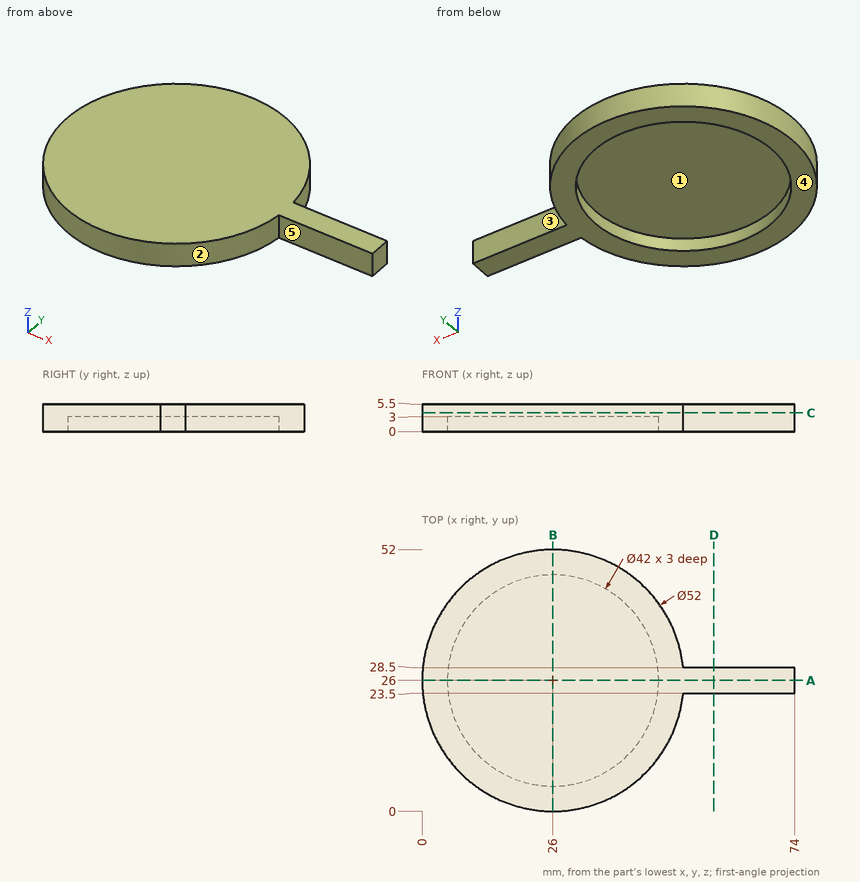
Design review of the part shown in the three views and the two pictorial views. Dimensions are in mm from the part's minimum x, y and z. A direction names the side the tool comes from. Coordinates: 2 decimals unless noted, no trailing zeros. Loops run counter-clockwise (first coordinate to the right, second up) from the corner with the lowest first, then second, coordinate; pieces in that order, holes last.
Q1. We need section D-D on x = 58. State the section outline as (y, z) points.
Reported:
outline: (23.5, 0) - (28.5, 0) - (28.5, 5.5) - (23.5, 5.5) - close
Q2. For pin 1 (10 mm diameter, centred on x = 35.5, y = 19.5, fed in from -Z); pin 2 (3 mm diameter, centred on x = 58.5, z = 2.5, fed in from +Y); pin 3 (1 mm diameter, centred on x = 19, z = 5, fed in from -Y), all flat-tipped, find the tip position at first contact; note any pin that passes through.
Reported:
pin 1: stops at z = 3
pin 2: stops at y = 28.5
pin 3: stops at y = 0.83
Q3. We need section B-B on x = 26. State the section outline as (y, z) points.
Reported:
outline: (0, 0) - (5, 0) - (5, 3) - (47, 3) - (47, 0) - (52, 0) - (52, 5.5) - (0, 5.5) - close
Q4. Tool access review of the marked faces 4 and 5: name each direction out of +Z, -Z, +X, -X, +Y, -Y from which nothing blocks a thin tool from reaching the whole face with its end or side.
Reported:
face 4: -Z, +X, -X, +Y, -Y
face 5: +Z, -Z, +X, -Y
Q5. We need section C-C on z = 3.75. State the section outline as (x, y) points.
Reported:
outline: (51.88, 23.5) - (74, 23.5) - (74, 28.5) - (51.88, 28.5) arc R26 ccw (long way) to start
Q6. We need section A-A on y = 26. State the section outline as (x, z) points, and give its area (3 significant figures).
Reported:
outline: (0, 0) - (5, 0) - (5, 3) - (47, 3) - (47, 0) - (74, 0) - (74, 5.5) - (0, 5.5) - close
area: 281 mm2
Q7. The part is to be moulded in two halves that separate along X. For the marked faces 1, 2 and 3, say which applies: +X half, -X half, draft (parallel to the pull), parting line (faces both ways), or undercut.
Reported:
face 1: undercut
face 2: parting line
face 3: draft
Q8. To check wall thickness, follow line 1 (X direction, y = 26, z = 1.25); line 2 (Y direction, x = 26, z = 2.2); line 3 (Y direction, x = 63.5, z = 4.5). State the ranges of each line that lie inside material, in increasing order.
Reported:
line 1: x = 0 to 5, 47 to 74
line 2: y = 0 to 5, 47 to 52
line 3: y = 23.5 to 28.5
